Work out the finished part from the listing and answer in its coordinate system (mm). A direction names the side the tool comes from. Give positions to 0.01 mm unless a question says otherwise; leave off trailing zeros. Write each loop counter-clockwise with the first axis right and the second up, starting at its lowest first coordinate (ties: lowest second). Pieces come first, ordered by that corner, then holes. Notation, with made-up numbers: (43.25, -7) -> (51.25, -7) arc R27 cw to (51.25, 30) -> close; hole circle Ø4 at (35.5, 43.25). An arc over 180 degrees is marked (long way). Write item = value, one per line. Start each with the question number.
from build123d import *

# Parameters (mm, degrees)
SKETCH7_W               = 86
SKETCH7_H               = 4
CUT_EXTRUDE3_DEPTH      = 122.688125961
CUT_EXTRUDE3_DEPTH_BACK = 122.688125961
SKETCH9_R               = 40
CUT_EXTRUDE4_DEPTH      = 122.688125961
SKETCH10_R              = 40
BOSS_EXTRUDE1_DEPTH     = 20
CUT_EXTRUDE7_DEPTH      = 124.255831505
CUT_EXTRUDE8_DEPTH      = 140.597641687
CUT_EXTRUDE8_DEPTH_BACK = 140.597641687
SKETCH15_R              = 3


with BuildPart() as part:
    # Sketch7 → Revolve4 (revolve)
    with BuildSketch(Plane.XY):
        with Locations((-43, -2)):
            Rectangle(SKETCH7_W, SKETCH7_H)
    revolve(axis=Axis((0, 0, 0), (0, -1, 0)))

    # Sketch9 → Cut-Extrude3 (cut, two sides: drawn at the far end of the back side and taken through both)
    with BuildSketch(Plane(origin=(0, 0, 0), x_dir=(1, 0, 0), z_dir=(0, 1, 0)).offset(-CUT_EXTRUDE3_DEPTH_BACK)):
        with Locations(Location((0, 0, 0), (0, 0, 270))):
            Circle(SKETCH9_R)
    extrude(amount=CUT_EXTRUDE3_DEPTH + CUT_EXTRUDE3_DEPTH_BACK, mode=Mode.SUBTRACT)

    # Sketch1 → Cut-Extrude4 (cut, through all)
    with BuildSketch(Plane(origin=(0, 0, 0), x_dir=(1, 0, 0), z_dir=(0, 1, 0))):
        with BuildLine():
            Line((-86.191983256, -25.902548569), (-9.566772234, -1.00550828))
            Line((-9.566772234, -1.00550828), (-89.693924294, 7.416194762))
            ThreePointArc((-89.693924294, 7.416194762), (-89.506970583, -9.407561694), (-86.191983256, -25.902548569))
        make_face()
    extrude(amount=-CUT_EXTRUDE4_DEPTH, mode=Mode.SUBTRACT)

    # Sketch10 → Boss-Extrude1 (add)
    with BuildSketch(Plane(origin=(0, 0, 0), x_dir=(-1, 0, 0), z_dir=(0, -1, 0))):
        with Locations(Location((0, 0, 0), (0, 0, 3.134016017))):
            Circle(SKETCH10_R)
    extrude(amount=BOSS_EXTRUDE1_DEPTH)

    # Sketch14 → Cut-Extrude7 (cut, through all)
    with BuildSketch(Plane(origin=(0, 0, 0), x_dir=(1, 0, 0), z_dir=(0, 1, 0))):
        Polygon((18.244865358, 22.530532352), (-22.530532352, 18.244865358), (-18.244865358, -22.530532352), (22.530532352, -18.244865358), align=None)
    extrude(amount=-CUT_EXTRUDE7_DEPTH, mode=Mode.SUBTRACT)

    # Sketch15 → Cut-Extrude8 (cut, two sides: drawn at the far end of the back side and taken through both)
    with BuildSketch(Plane(origin=(-2.142833497, 0, -20.387698855), x_dir=(0.9945218953682733, 0, -0.10452846326765386), z_dir=(0.10452846326765386, 0, 0.9945218953682733)).offset(-CUT_EXTRUDE8_DEPTH_BACK)):
        with Locations((0, -10)):
            Circle(SKETCH15_R)
    extrude(amount=CUT_EXTRUDE8_DEPTH + CUT_EXTRUDE8_DEPTH_BACK, mode=Mode.SUBTRACT)


solid = part.part
(1) Find the intervals of material crossed by line 1 along Y through (x, z) = (69, 50); line 2 along X through (y, z) = (-12.75, 18); line 3 along X through (y, z) = (-10, -32.5), in increasing order.
(2) Determine the mould class of faces 5 (the cylindrical face through (0.95, -7.97, 30.18)), 6 (the flat face through (-16.2, -20, -19.3)), 7 (the flat face through (-1.857, -5.416, -20.418)), 8 (the flat face through (19, 0, 19)) for opening direction Y: pulls with the +Y half, pulls with the -Y half, needs draft (parallel to the pull), parting line crosses it, or undercut.
(3) A cutting plane is placed at C-C, the plane x = -35. Write down the section's boundary in (y, z).
(4) A cutting plane is placed at D-D, the plane z = 58.5. Write down the section's boundary in (x, y).
(5) A cutting plane is placed at B-B, the plane z = 0. Write down the section's boundary in (x, y).
(6) For faces 1 (the cylindrical face through (-19.63, -12.08, -34.85)), 2 (the cylindrical face through (-1.57, -7.47, -30.39)), 3 (the flat face through (-62.51, -1.97, -4.56)), 4 (the flat face through (-20.418, -9.86, 1.857)), determine the directions among +Z, -Z, +X, -X, +Y, -Y from which every point of the face is accessible in a straight line to the end or side of a thin tool.
(7) Each of these flat-tipped pins is pushed along its axis until it touches: pin 1 (1.5 mm diameter, centred on y = -8, z = 32, fed in from -X); pin 2 (3 mm diameter, centred on x = 47, y = -3, fed in from -Z); pin 3 (2 mm diameter, centred on x = 13.5, y = -13, fed in from +Z). Where does it stop, or does it pass through?
(8) A cutting plane is placed at A-A, the plane y = -15. Write down the section's boundary in (x, z), then the cut area to 3 significant figures.
Results list:
q1.line_1 = -4 to 0
q1.line_2 = -35.72 to -18.72, 22.5 to 35.72
q1.line_3 = -23.32 to -6.43, -0.4 to 23.32
q2.face_5 = undercut
q2.face_6 = pulls with the -Y half
q2.face_7 = needs draft
q2.face_8 = pulls with the +Y half
q3.outline = (-20, -19.36) -> (-4, -19.36) -> (-4, -78.56) -> (0, -78.56) -> (0, 78.56) -> (-4, 78.56) -> (-4, 19.36) -> (-20, 19.36) -> close
q4.outline = (-63.04, -4) -> (63.04, -4) -> (63.04, 0) -> (-63.04, 0) -> close
q5.outline = (-40, -20) -> (-20.61, -20) -> (-20.61, 0) -> (-40, 0) -> close; (20.61, -20) -> (40, -20) -> (40, -4) -> (86, -4) -> (86, 0) -> (20.61, 0) -> close
q6.face_1 = -Y
q6.face_2 = none
q6.face_3 = -X, +Y, -Y
q6.face_4 = +Y, -Y
q7.pin_1 = -24.97
q7.pin_2 = -72.98
q7.pin_3 = 38
q8.outline = circle Ø80 at (0, 0); hole (-22.53, -18.24) -> (18.24, -22.53) -> (22.53, 18.24) -> (-18.24, 22.53) -> close
q8.area = 3,350 mm²
